The figure shows three views and two pictorial views of one solid part (mm, origin at its lowest corner). Answer the questions. A direction names the side the tool comes from. Coordinates: 2 decimals unless noted, no trailing zeros. Loops run counter-clockwise (first coordinate to the right, second up) from the corner with the lowest first, then second, coordinate; pieces in that order, holes last. Notation, with made-up numbers: (-8.5, -7) -> (12.5, -7) arc R33 ccw to (12.5, 23) -> close; hole circle Ø8 at (78, 26). An arc over 180 degrees is marked (long way). Answer in a Markdown table with one row per item.
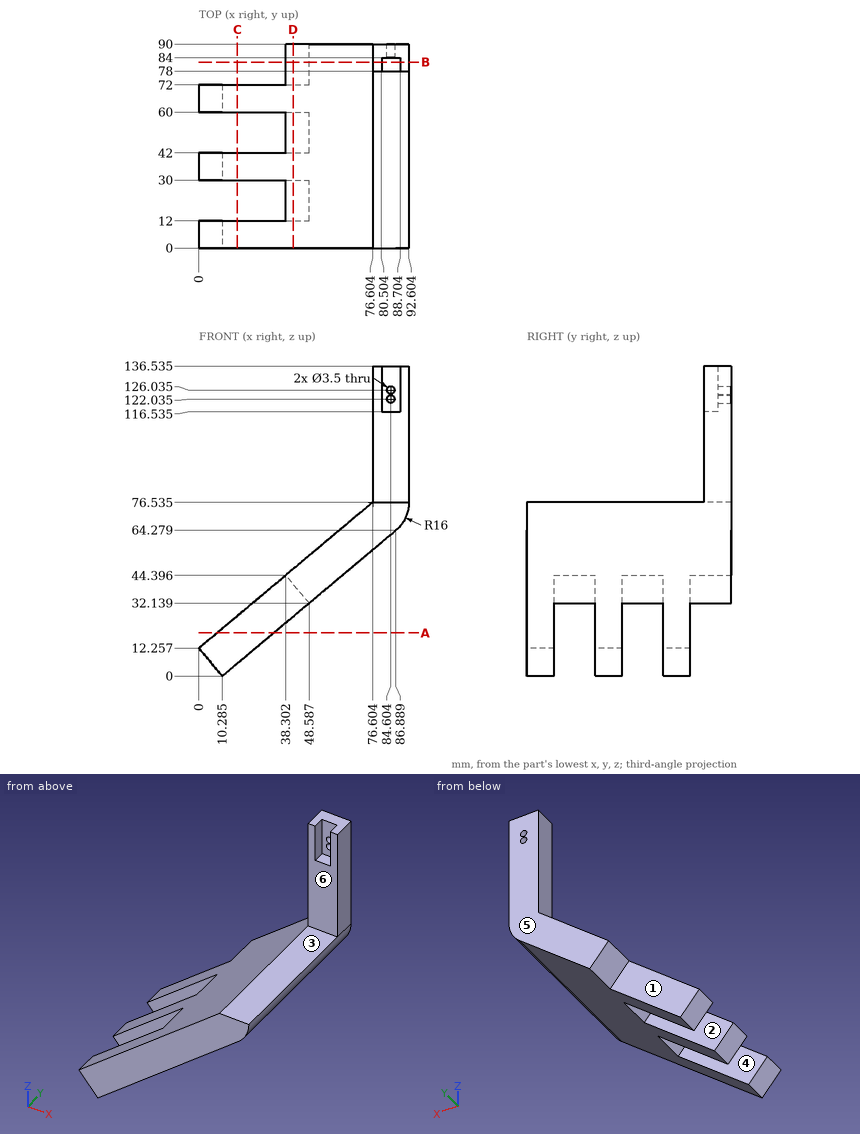
Item 1: Determine the mould class of the marked faces 4, 5 and 6 for opening direction Y: +Y half, -Y half, draft (parallel to the pull), parting line (faces both ways), or undercut.
Findings below:
| item | result |
|---|---|
| face 4 | undercut |
| face 5 | +Y half |
| face 6 | -Y half |
Item 2: A cutting plane is placed at A-A, the plane z = 19. Determine the outline of the cut face in (x, y).
Findings below:
| item | result |
|---|---|
| outline | (8.04, 0) -> (32.93, 0) -> (32.93, 12) -> (8.04, 12) -> close; (8.04, 30) -> (32.93, 30) -> (32.93, 42) -> (8.04, 42) -> close; (8.04, 60) -> (32.93, 60) -> (32.93, 72) -> (8.04, 72) -> close |
Item 3: A cutting plane is placed at B-B, the plane y = 82. Determine the outline of the cut face in (x, z) (1 decimal), plus the area to 3 significant figures.
Findings below:
| item | result |
|---|---|
| outline | (38.3, 44.4) -> (48.6, 32.1) -> (86.9, 64.3) arc R16 ccw to (92.6, 76.5) -> (92.6, 136.5) -> (88.7, 136.5) -> (88.7, 116.5) -> (80.5, 116.5) -> (80.5, 136.5) -> (76.6, 136.5) -> (76.6, 76.5) -> close |
| area | 1,710 mm2 |
Item 4: A cutting plane is placed at D-D, the plane x = 41.5. Determine the outline of the cut face in (y, z) (1 decimal), plus the area to 3 significant figures.
Findings below:
| item | result |
|---|---|
| outline | (0, 26.2) -> (12, 26.2) -> (12, 40.6) -> (30, 40.6) -> (30, 26.2) -> (42, 26.2) -> (42, 40.6) -> (60, 40.6) -> (60, 26.2) -> (72, 26.2) -> (72, 40.6) -> (90, 40.6) -> (90, 47.1) -> (0, 47.1) -> close |
| area | 1,100 mm2 |
Item 5: A cutting plane is placed at C-C, the plane x = 17. Determine the outline of the cut face in (y, z) (1 decimal), plus the area to 3 significant figures.
Findings below:
| item | result |
|---|---|
| outline | (0, 5.6) -> (12, 5.6) -> (12, 26.5) -> (0, 26.5) -> close; (30, 5.6) -> (42, 5.6) -> (42, 26.5) -> (30, 26.5) -> close; (60, 5.6) -> (72, 5.6) -> (72, 26.5) -> (60, 26.5) -> close |
| area | 752 mm2 |
Item 6: A tool of negligible diameter and unlimited length cuts with its end or side. For the marked faces 1, 2 and 3, from which of +Z, -Z, +X, -X, +Y, -Y can it reach the whole face along a straight path? Write none if from no direction.
Findings below:
| item | result |
|---|---|
| face 1 | -Z, -X, +Y |
| face 2 | -Z, -X |
| face 3 | +Z, +X, -X, -Y |
Item 7: Flat-ended cylindrical pins translate along their axes: pin 1 Ø2 at (x, y) = (55, 60.5) entering from -Z; pin 2 Ø4 at (y, z) = (59, 18) entering from +X; pin 3 Ø4 at (x, z) = (83.5, 124.5) entering from -Y; pin 4 Ø13.5 at (x, z) = (27.5, 33) entering from -Y. Find the tip coordinate at first contact, or state that the pin passes through.
Findings below:
| item | result |
|---|---|
| pin 1 | stops at z = 36.68 |
| pin 2 | stops at x = 33.8 |
| pin 3 | stops at y = 84 |
| pin 4 | stops at y = 0 |
Item 8: Find the intervals of material crossed by probe 1 along X at (y, z) = (83.5, 125) (1 decimal); probe 2 along Z at (x, y) = (78.5, 13.5) (1 decimal); probe 3 along X at (y, z) = (79.5, 105) (1 decimal), in increasing order.
Findings below:
| item | result |
|---|---|
| probe 1 | x = 76.6 to 80.5, 88.7 to 92.6 |
| probe 2 | z = 57.2 to 76.5 |
| probe 3 | x = 76.6 to 92.6 |
